Autodesk Inventor part; units mm, degrees
ref_plane "YZ Plane" through (0, 0, 0) normal (1, 0, 0) x (0, 1, 0)
ref_plane "XZ Plane" through (0, 0, 0) normal (0, 1, 0) x (-1, 0, 0)
ref_plane "XY Plane" through (0, 0, 0) normal (0, 0, 1) x (1, 0, 0)
sketch "Sketch1" plane through (0, 0, 0) normal (0, 0, 1) x (1, 0, 0)
  line L0 (-571.5, -609.6) -> (571.5, -609.6)
  line L1 (571.5, -609.6) -> (571.5, 609.6)
  line L2 (571.5, 609.6) -> (-571.5, 609.6)
  line L3 (-571.5, 609.6) -> (-571.5, -609.6)
  line L4 (-571.5, -609.6) -> (571.5, 609.6) construction
  line L5 (571.5, -609.6) -> (-571.5, 609.6) construction
  line L6 (-30.4012, 32.4279) -> (30.4012, -32.4279)
  line L7 (-510.6976, -609.6) -> (571.5, 544.7441)
  line L8 (-571.5, -544.7441) -> (510.6976, 609.6)
  point P0 (0, 0)
  point P1 (474.8791, 609.6)
  dimension "d6" = 88.9
extrude "Extrusion1" add sketch "Sketch1" along normal blind 38.1 contours L3 L8 L6 L7 L0 | L6 L8 L2 L1 L7
properties part number "S_2x4x65.795"
Part model, mm, in its own coordinate system. Give positions to 0.01 mm unless a question says otherwise; leave off trailing zeros. Order: outer loops, then holes, each group sorted by start corner. A loop starts at its lowest first (then second) coordinate and runs counter-clockwise, first axis right, second up. Notation, with made-up numbers: M -28.5,-22.5 L 7.5,-22.5 A20 cw 7.5,-17.5 Z; hole C 81,-4 d5. An arc over 180 degrees is marked long. Use a Markdown table: item, result. Add a question column.
(1) Probe line 1 along X through (y, z) = (-272, 34.5); line 2 along Y through (x, z) = (-98, 32); line 3 along X through (y, z) = (-25, 27.5). List the from-to ranges inside material, lowest first. Write a range as [from, to].
(2) Saw through at B-B, the plane y = 298.5. Give the cut face in (x, z).
(3) Drop flat-ended pins along their axis: P1, Ø4, axis at y = 424, z = 20.5, coming from the +X side; P2, Ø4, axis at y = 403.5, z = 22.5, coming from the -X side; P3, Ø4, axis at x = -39.5, z = 17, coming from the +Y side. Give the stop position or say it passes through.
(4) Saw through at C-C, the plane x = -88.5. Give the cut face in (y, z).
(5) Saw through at A-A, the plane z = 10.5. Give the cut face in (x, y), and give its area (3 significant figures).
Answer key:
| question | item | result |
|---|---|---|
| 1 | line 1 | [-315.8, -194.2] |
| 1 | line 2 | [-169.39, -39.68] |
| 1 | line 3 | [-84.24, 37.36] |
| 2 | outline | M 219.04,0 L 340.65,0 L 340.65,38.1 L 219.04,38.1 Z |
| 3 | P1 | x = 460.18 |
| 3 | P2 | x = 315.6 |
| 3 | P3 | y = 24.86 |
| 4 | outline | M -159.26,0 L -29.54,0 L -29.54,38.1 L -159.26,38.1 Z |
| 5 | outline | M -571.5,-609.6 L -510.7,-609.6 L 571.5,544.74 L 571.5,609.6 L 510.7,609.6 L -571.5,-544.74 Z |
| 5 | area | 144,000 mm^2 |
